Read the model definition and answer for the solid it produces. Units are mm, in the model's axes. A direction names the side the tool comes from. Coordinates: 2 decimals unless noted, no trailing zeros. Order: outer loops, then holes, each group sorted by start corner. A loop starts at its lowest first (then second) coordinate and runs counter-clockwise, first axis right, second up.
```python
from build123d import *

# Parameters (mm, degrees)
SKETCH1_W           = 20
SKETCH1_H           = 50
BOSS_EXTRUDE1_DEPTH = 4.45
SKETCH2_W           = 45
SKETCH2_H           = 40
BOSS_EXTRUDE2_DEPTH = 5
CUT_EXTRUDE1_REACH  = 75.824
SKETCH4_R           = 2.75
SKETCH5_R           = 2.75
CUT_EXTRUDE2_DEPTH  = 72.199034404
SKETCH6_W           = 4.45
SKETCH6_H           = 20
BOSS_EXTRUDE3_DEPTH = 23
SKETCH7_R           = 2.75
CUT_EXTRUDE3_DEPTH  = 91.157098999
BOSS_EXTRUDE4_DEPTH = 3
BOSS_EXTRUDE5_DEPTH = 3


with BuildPart() as part:
    # Sketch1 → Boss-Extrude1 (new body)
    with BuildSketch(Plane(origin=(0, 0, 0), x_dir=(0, 0, -1), z_dir=(1, 0, 0))):
        with Locations((10, 25)):
            Rectangle(SKETCH1_W, SKETCH1_H)
    extrude(amount=BOSS_EXTRUDE1_DEPTH)

    # Sketch2 → Boss-Extrude2 (add)
    with BuildSketch(Plane(origin=(0, 50, 0), x_dir=(1, 0, 0), z_dir=(0, 1, 0))):
        with Locations((22.5, 0)):
            Rectangle(SKETCH2_W, SKETCH2_H)
    extrude(amount=BOSS_EXTRUDE2_DEPTH)

    # Sketch4 → Cut-Extrude1 (cut, up to next)
    with BuildSketch(Plane(origin=(0, 55, 0), x_dir=(1, 0, 0), z_dir=(0, 1, 0)), mode=Mode.PRIVATE) as cut_extrude1_sk1:
        with Locations(Location((32.25, -0.85, 0), (0, 0, 270))):
            Circle(SKETCH4_R)
    cut_extrude1_tool1 = extrude(cut_extrude1_sk1.sketch, amount=-CUT_EXTRUDE1_REACH, mode=Mode.PRIVATE) & part.part
    # Sketch4 → Cut-Extrude1 (cut, up to next)
    with BuildSketch(Plane(origin=(0, 55, 0), x_dir=(1, 0, 0), z_dir=(0, 1, 0)), mode=Mode.PRIVATE) as cut_extrude1_sk2:
        with Locations(Location((16.2, 10.75, 0), (0, 0, 270))):
            Circle(SKETCH4_R)
    cut_extrude1_tool2 = extrude(cut_extrude1_sk2.sketch, amount=-CUT_EXTRUDE1_REACH, mode=Mode.PRIVATE) & part.part
    add(cut_extrude1_tool1.solids().sort_by_distance((32.25, 55, 0.85))[0], mode=Mode.SUBTRACT)
    add(cut_extrude1_tool2.solids().sort_by_distance((16.2, 55, -10.75))[0], mode=Mode.SUBTRACT)

    # Sketch5 → Cut-Extrude2 (cut, through all)
    with BuildSketch(Plane(origin=(4.45, 0, 0), x_dir=(0, 0, -1), z_dir=(1, 0, 0))):
        with Locations((9, 24)):
            Circle(SKETCH5_R)
        with Locations((5.5, 7)):
            Circle(SKETCH5_R)
    extrude(amount=-CUT_EXTRUDE2_DEPTH, mode=Mode.SUBTRACT)

    # Sketch6 → Boss-Extrude3 (add)
    with BuildSketch(Plane(origin=(0, 55, 0), x_dir=(1, 0, 0), z_dir=(0, 1, 0))):
        with Locations((2.225, 10)):
            Rectangle(SKETCH6_W, SKETCH6_H)
    extrude(amount=BOSS_EXTRUDE3_DEPTH)

    # Sketch7 → Cut-Extrude3 (cut, through all)
    with BuildSketch(Plane(origin=(4.45, 0, 0), x_dir=(0, 0, -1), z_dir=(1, 0, 0))):
        with Locations((8.3, 67.9)):
            Circle(SKETCH7_R)
    extrude(amount=-CUT_EXTRUDE3_DEPTH, mode=Mode.SUBTRACT)

    # Sketch8 → Boss-Extrude4 (add)
    with BuildSketch(Plane(origin=(0, 0, -20), x_dir=(-1, 0, 0), z_dir=(0, 0, -1))):
        Polygon((-4.45, 78), (-4.45, 55), (-45, 55), align=None)
    extrude(amount=-BOSS_EXTRUDE4_DEPTH)

    # Sketch9 → Boss-Extrude5 (add)
    with BuildSketch(Plane.XY):
        Polygon((4.45, 55), (24.45, 55), (4.45, 78), (0, 78), (0, 55), align=None)
    extrude(amount=BOSS_EXTRUDE5_DEPTH)


solid = part.part
```
1) Which of the six approach directions +Z, -Z, +X, -X, +Y, -Y give full straight-line access (tool end or side, diameter ignored) to faces 1 (the flat face through (4.45, 25, -12)), 2 (the flat face through (14.59, 66.34, 1.48)), 3 (the flat face through (2, 25, 0)), 4 (the flat face through (15, 62, -17))?
A:
face 1: +Z, -Z, +X, -Y
face 2: +Z, +X, +Y
face 3: +Z, +X, -X, -Y
face 4: +X, +Y
2) A cutting plane is placed at A-A, the plane y = 24. Determine the outline of the cut face in (x, z).
A:
outline: (0, -20) - (4.45, -20) - (4.45, -11.75) - (0, -11.75) - close; (0, -6.25) - (4.45, -6.25) - (4.45, 0) - (0, 0) - close
3) Determine the mould class of faces 5 (the cylindrical face through (2.26, 4.56, -6.77)), 6 (the cylindrical face through (2.256, 26.727, -8.642)), 7 (the flat face through (10, 62, 0)), 8 (the flat face through (27, 55, 1)) for opening direction Y: pulls with the +Y half, pulls with the -Y half, needs draft (parallel to the pull), parting line crosses it, or undercut.
A:
face 5: undercut
face 6: undercut
face 7: needs draft
face 8: pulls with the +Y half
4) A cutting plane is placed at B-B, the plane z = 0.85. Determine the outline of the cut face in (x, y).
A:
outline: (0, 50) - (29.5, 50) - (29.5, 55) - (24.45, 55) - (4.45, 78) - (0, 78) - close; (35, 50) - (45, 50) - (45, 55) - (35, 55) - close
5) A cutting plane is placed at D-D, the plane y = 58. Determine the outline of the cut face in (x, z), and give its area (3 significant figures).
A:
outline: (0, -20) - (39.71, -20) - (39.71, -17) - (4.45, -17) - (4.45, 0) - (21.84, 0) - (21.84, 3) - (0, 3) - close
area: 260 mm2
6) Flat-ended cylindrical pins translate along their axes: pin 1 Ø9 at (y, z) = (7, -5.5) entering from +X; pin 2 Ø7 at (x, y) = (12, 64.5) entering from +Z; pin 3 Ø9 at (x, z) = (32.25, 0.85) entering from +Y; pin 4 Ø8 at (y, z) = (57.5, -14) entering from +X. Find the tip coordinate at first contact, or state that the pin passes through.
A:
pin 1: stops at x = 4.45
pin 2: stops at z = 3
pin 3: stops at y = 55
pin 4: stops at x = 45
7) Straight lines are drawn through the part: line 1 (Z direction, x = 16, y = 52); line 2 (Y direction, x = 3.4, z = -5.5); line 3 (X direction, y = 51.45, z = 0.85). For each, find the intervals that lie inside material, in ascending order.
A:
line 1: z = -20 to -13.49, -8.01 to 20
line 2: y = 0 to 4.25, 9.75 to 78
line 3: x = 0 to 29.5, 35 to 45
8) A cutting plane is placed at C-C, the plane x = 16.2. Determine the outline of the cut face in (y, z).
A:
outline: (50, -20) - (71.34, -20) - (71.34, -17) - (55, -17) - (55, -13.5) - (50, -13.5) - close; (50, -8) - (55, -8) - (55, 0) - (64.49, 0) - (64.49, 3) - (55, 3) - (55, 20) - (50, 20) - close
